Read the model definition and answer for the solid it produces. Units are mm, in the model's axes. Face numbers are marked on the shaded views. A direction names the side the tool comes from. Coordinates: 2 decimals unless noted, no trailing zeros. Write each loop counter-clockwise with the first axis right and the second up, starting at its lowest first coordinate (ties: lowest second). Pieces come first, ordered by that corner, then holes.
1) Find the intervals of material crossed by line 1 (Z direction, x = 0.5, y = 0); line 2 (Y direction, x = 4.25, z = 9.5); line 3 (Y direction, x = 7.5, z = 10.5), in increasing order.
2) The part is cut by section D-D (z = 13). Determine the outline of the cut face in (x, y).
3) The part is cut by section B-B (y = 0). Determine the outline of the cut face in (x, z), then the cut area to 3 significant figures.
4) Determine the mould class of the marked faces 1, 2 and 3 for opening direction Y: +Y half, -Y half, draft (parallel to the pull), parting line (faces both ways), or undercut.
5) The part is cut by section A-A (z = 0). Determine the outline of the cut face in (x, y).
6) Each of these flat-tipped pins is pushed along its axis until it touches: pin 1 Ø1 at (x, y) = (6.5, 19) entering from -Z; pin 2 Ø4 at (x, y) = (4.5, -11.5) entering from +Z; pin 3 Ø4.5 at (x, z) = (4, -0.5) entering from +Y; pin 4 Ø1 at (x, y) = (1.5, -5.5) entering from +Z. Where does it stop, or does it pass through?
7) The part is cut by section C-C (x = 5.25). Determine the outline of the cut face in (y, z), then the cut area to 3 significant figures.
8) Which of the six approach directions +Z, -Z, +X, -X, +Y, -Y give full straight-line access (tool end or side, diameter ignored) to the marked faces 4, 5 and 6?
from build123d import *

# Parameters (mm, degrees)
F0_R     = 25.1
F1_DEPTH = 8
F3_DEPTH = 7
F4_R     = 1.5
F5_DEPTH = 25
F6_W     = 5
F6_H     = 2.87


with BuildPart() as f1:
    # F0 (on Right) → F1 (new body)
    with BuildSketch(Plane.YZ):
        Circle(F0_R)
        with BuildLine():
            ThreePointArc((-3.277508, -19.802201), (-14.192766, -14.192766), (-19.802201, -3.277508))
            Line((-19.802201, -3.277508), (-3.277508, -3.277508))
            Line((-3.277508, -3.277508), (-3.277508, -19.802201))
        make_face(mode=Mode.SUBTRACT)
        with BuildLine():
            ThreePointArc((19.802201, -3.277508), (14.192766, -14.192766), (3.277508, -19.802201))
            Line((3.277508, -19.802201), (3.277508, -3.277508))
            Line((3.277508, -3.277508), (19.802201, -3.277508))
        make_face(mode=Mode.SUBTRACT)
        with BuildLine():
            ThreePointArc((-19.802201, 3.277508), (-14.192766, 14.192766), (-3.277508, 19.802201))
            Line((-3.277508, 19.802201), (-3.277508, 3.277508))
            Line((-3.277508, 3.277508), (-19.802201, 3.277508))
        make_face(mode=Mode.SUBTRACT)
        with BuildLine():
            Line((3.277508, 3.277508), (3.277508, 19.802201))
            ThreePointArc((3.277508, 19.802201), (14.192766, 14.192766), (19.802201, 3.277508))
            Line((19.802201, 3.277508), (3.277508, 3.277508))
        make_face(mode=Mode.SUBTRACT)
    extrude(amount=F1_DEPTH)

    # F2 (on face) → F3 (cut)
    with BuildSketch(Plane.YZ.offset(8)):
        with BuildLine():
            Line((-2.4, 1.962142), (-2.4, -1.962142))
            ThreePointArc((-2.4, -1.962142), (0, -3.1), (2.4, -1.962142))
            Line((2.4, -1.962142), (2.4, 1.962142))
            ThreePointArc((2.4, 1.962142), (0, 3.1), (-2.4, 1.962142))
        make_face()
    extrude(amount=-F3_DEPTH, mode=Mode.SUBTRACT)

    # F4 (on face) → F5 (cut)
    with BuildSketch(Plane.YZ.offset(1)):
        Circle(F4_R)
    extrude(amount=-F5_DEPTH, mode=Mode.SUBTRACT)

    # F6 (on Top) → F7 (revolve)
    with BuildSketch(Plane.XY):
        with Locations((4, 26.535)):
            Rectangle(F6_W, F6_H)
    revolve(axis=Axis((8, 0, 0), (1, 0, 0)))


solid = f1.part
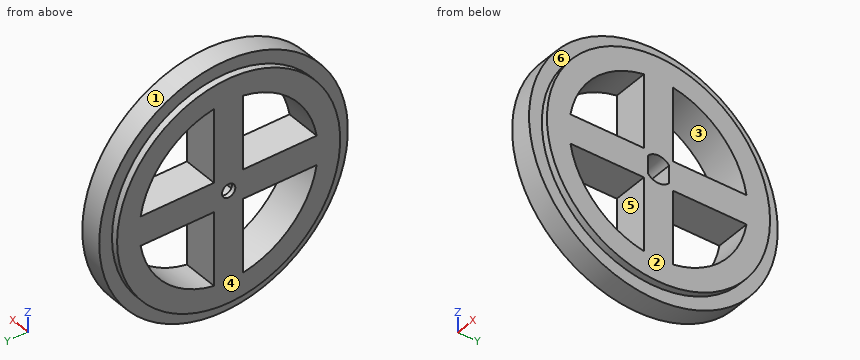
Reported:
1. line 1: z = -25.1 to -1.5, 1.5 to 25.1
1. line 2: y = -26.31 to -17.68, -3.28 to 3.28, 17.68 to 26.31
1. line 3: y = -22.8 to -17.11, -3.28 to 3.28, 17.11 to 22.8
2. outline: (0, -21.47) - (1.5, -21.47) - (1.5, -24.77) - (6.5, -24.77) - (6.5, -21.47) - (8, -21.47) - (8, -15.29) - (0, -15.29) - close; (0, -3.28) - (8, -3.28) - (8, 3.28) - (0, 3.28) - close; (0, 15.29) - (8, 15.29) - (8, 21.47) - (6.5, 21.47) - (6.5, 24.77) - (1.5, 24.77) - (1.5, 21.47) - (0, 21.47) - close
3. outline: (0, -25.1) - (1.5, -25.1) - (1.5, -27.97) - (6.5, -27.97) - (6.5, -25.1) - (8, -25.1) - (8, -3.1) - (1, -3.1) - (1, -1.5) - (0, -1.5) - close; (0, 1.5) - (1, 1.5) - (1, 3.1) - (8, 3.1) - (8, 25.1) - (6.5, 25.1) - (6.5, 27.97) - (1.5, 27.97) - (1.5, 25.1) - (0, 25.1) - close
3. area: 384 mm2
4. face 1: parting line
4. face 2: draft
4. face 3: undercut
5. outline: (0, -25.1) - (1.5, -25.1) - (1.5, -27.97) - (6.5, -27.97) - (6.5, -25.1) - (8, -25.1) - (8, -2.4) - (1, -2.4) - (1, -1.5) - (0, -1.5) - close; (0, 1.5) - (1, 1.5) - (1, 2.4) - (8, 2.4) - (8, 25.1) - (6.5, 25.1) - (6.5, 27.97) - (1.5, 27.97) - (1.5, 25.1) - (0, 25.1) - close
6. pin 1: stops at z = -20.98
6. pin 2: stops at z = 26.31
6. pin 3: stops at y = 27.97
6. pin 4: stops at z = 27.52
7. outline: circle Ø55.94 at (0, 0); hole (-19.8, -3.28) arc R20.07 ccw to (-3.28, -19.8) - (-3.28, -3.28) - close; hole (-19.8, 3.28) - (-3.28, 3.28) - (-3.28, 19.8) arc R20.07 ccw to start; hole (-2.4, -1.96) arc R3.1 ccw to (2.4, -1.96) - (2.4, 1.96) arc R3.1 ccw to (-2.4, 1.96) - close; hole (3.28, -19.8) arc R20.07 ccw to (19.8, -3.28) - (3.28, -3.28) - close; hole (3.28, 3.28) - (19.8, 3.28) arc R20.07 ccw to (3.28, 19.8) - close
7. area: 1,650 mm2
8. face 4: +Z, -Z, -X, +Y, -Y
8. face 5: +X, -X
8. face 6: +X
